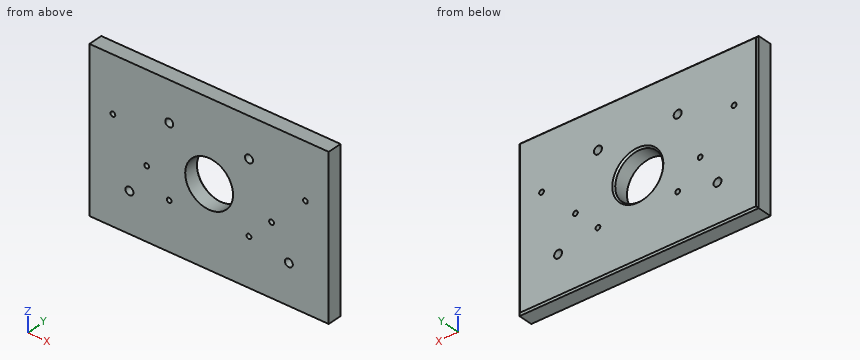
```python
from build123d import *

# Parameters (mm, degrees)
SKETCH1_W           = 150
SKETCH1_H           = 100
BOSS_EXTRUDE1_DEPTH = 10
SKETCH2_R           = 15
SKETCH2_R_2         = 1.5
SKETCH2_R_3         = 2.5
CUT_EXTRUDE1_DEPTH  = 181.554700853
CHAMFER1_SIZE       = 1


with BuildPart() as part:
    # Sketch1 → Boss-Extrude1 (new body)
    with BuildSketch(Plane(origin=(0, 0, 0), x_dir=(1, 0, 0), z_dir=(0, 1, 0))):
        with Locations((75, 50)):
            Rectangle(SKETCH1_W, SKETCH1_H)
    extrude(amount=BOSS_EXTRUDE1_DEPTH)

    # Sketch2 → Cut-Extrude1 (cut, through all)
    with BuildSketch(Plane(origin=(0, 10, 0), x_dir=(1, 0, 0), z_dir=(0, 1, 0))):
        with Locations(Location((75, 50, 0), (0, 0, 270))):
            Circle(SKETCH2_R)
        with Locations(Location((100, 70, 0), (0, 0, 90))):
            Circle(SKETCH2_R_2)
        with Locations(Location((125, 75, 0), (0, 0, 90))):
            Circle(SKETCH2_R_3)
        with Locations(Location((114.142135624, 55.857864376, 0), (0, 0, 90))):
            Circle(SKETCH2_R_2)
        with Locations(Location((135.355339059, 34.644660941, 0), (0, 0, 90))):
            Circle(SKETCH2_R_2)
        with Locations(Location((100, 25, 0), (0, 0, 90))):
            Circle(SKETCH2_R_3)
        with Locations(Location((50, 25, 0), (0, 0, 270))):
            Circle(SKETCH2_R_3)
        with Locations(Location((14.644660941, 34.644660941, 0), (0, 0, 270))):
            Circle(SKETCH2_R_2)
        with Locations(Location((35.857864376, 55.857864376, 0), (0, 0, 270))):
            Circle(SKETCH2_R_2)
        with Locations(Location((50, 70, 0), (0, 0, 270))):
            Circle(SKETCH2_R_2)
        with Locations(Location((25, 75, 0), (0, 0, 270))):
            Circle(SKETCH2_R_3)
    extrude(amount=-CUT_EXTRUDE1_DEPTH, mode=Mode.SUBTRACT)

    # Chamfer1
    chamfer1_edges = [part.edges().sort_by_distance(p)[0] for p in [
        (150, 10, -50),
        (75, 10, -100),
        (75, 10, -65),
        (0, 10, -50),
        (75, 10, 0),
    ]]
    chamfer(chamfer1_edges, length=CHAMFER1_SIZE)


solid = part.part
```
Check sheet for the modelled part. Datum: model origin and axes. Units: mm. Round coordinates to 2 decimals unless told otherwise and drop trailing zeros. Loops run counter-clockwise (first coordinate to the right, second up) from the corner with the lowest first, then second, coordinate; pieces in that order, holes last. Notation, with made-up numbers: (62.25, -18.75) - (74.25, -18.75) arc R30 ccw to (74.25, 16.25) - close; hole circle Ø5 at (38.25, 49). An arc over 180 degrees is marked (long way). Answer as a JSON object with one key per item and string values. Group by question number.
Q1. Gauge pin test, flat ends, axial feed: P1, Ø8, axis at x = 25, z = -75, coming from the -Y side; P2, Ø2.5, axis at x = 135.36, z = -34.64, coming from the -Y side. Record the tip position at first contact, or that the pin passes through.
Q2. Scan lines: line 1 along X through (y, z) = (4.5, -25); line 2 along X through (y, z) = (2.5, -70); line 3 along Z through (x, y) = (100, 1). Record each from-to range of solid material in increasing order. Write a range as [from, to].
Q3. Sectioned sample at D-D, the plane z = -50. Enter the section's corners in (x, y), plus the area to 3 significant figures.
Q4. Sectioned sample at B-B, the plane z = -75. Enter the section's corners in (x, y), plus the area to 3 significant figures.
Q5. Sectioned sample at A-A, the plane x = 75. Enter the section's corners in (y, z).
Q6. Sectioned sample at C-C, the plane x = 50. Enter the section's corners in (y, z), plus the area to 3 significant figures.
Solution:
{
 "1": {"P1": "stops at y = 0", "P2": "passes through"},
 "2": {"line 1": "x = [0, 47.5], [52.5, 97.5], [102.5, 150]", "line 2": "x = [0, 48.5], [51.5, 98.5], [101.5, 150]", "line 3": "z = [-100, -71.5], [-68.5, -27.5], [-22.5, 0]"},
 "3": {"outline": "(0, 0) - (60, 0) - (60, 9) - (59, 10) - (1, 10) - (0, 9) - close; (90, 0) - (150, 0) - (150, 9) - (149, 10) - (91, 10) - (90, 9) - close", "area": "1,200 mm²"},
 "4": {"outline": "(0, 0) - (22.5, 0) - (22.5, 10) - (1, 10) - (0, 9) - close; (27.5, 0) - (122.5, 0) - (122.5, 10) - (27.5, 10) - close; (127.5, 0) - (150, 0) - (150, 9) - (149, 10) - (127.5, 10) - close", "area": "1,400 mm²"},
 "5": {"outline": "(0, -100) - (9, -100) - (10, -99) - (10, -66) - (9, -65) - (0, -65) - close; (0, -35) - (9, -35) - (10, -34) - (10, -1) - (9, 0) - (0, 0) - close"},
 "6": {"outline": "(0, -100) - (9, -100) - (10, -99) - (10, -71.5) - (0, -71.5) - close; (0, -68.5) - (10, -68.5) - (10, -27.5) - (0, -27.5) - close; (0, -22.5) - (10, -22.5) - (10, -1) - (9, 0) - (0, 0) - close", "area": "919 mm²"}
}
